from build123d import *

# Parameters (mm, degrees)
SKETCH1_W          = 12
SKETCH1_H          = 2.5
CHAMFER1_SIZE      = 0.6
CUT_EXTRUDE2_DEPTH = 1.925


with BuildPart() as part:
    # Sketch1 → Revolve1 (revolve)
    with BuildSketch(Plane(origin=(0, 0, 0), x_dir=(0, 0, -1), z_dir=(1, 0, 0))):
        with Locations((8.75, 1.25)):
            Rectangle(SKETCH1_W, SKETCH1_H)
    revolve(axis=Axis((0, 0, -14.75), (0, 0, 1)))

    # Chamfer1
    chamfer1_edges = [part.edges().sort_by_distance(p)[0] for p in [
        (0, -2.5, -14.75),
    ]]
    chamfer(chamfer1_edges, length=CHAMFER1_SIZE)

    # Sketch7 → Revolve2 (revolve)
    with BuildSketch(Plane(origin=(0, 0, 0), x_dir=(0, 0, -1), z_dir=(1, 0, 0)), mode=Mode.PRIVATE) as revolve2_sk:
        with BuildLine():
            Line((2.3375, 4.75), (2.75, 4.75))
            Line((2.75, 4.75), (2.75, 0))
            Line((2.75, 0), (0, 0))
            Line((0, 0), (0, 2.5))
            ThreePointArc((0, 2.5), (0.991875183, 3.808753282), (2.3375, 4.75))
        make_face()
    revolve(revolve2_sk.sketch.rotate(Axis((0, 0, 0), (0, 0, -1)), 180), axis=Axis((0, 0, 0), (0, 0, -1)))

    # Sketch5 → Cut-Extrude2 (cut)
    with BuildSketch(Plane.XY):
        Polygon((1.5, -0.866025404), (1.5, 0.866025404), (0, 1.732050808), (-1.5, 0.866025404), (-1.5, -0.866025404), (0, -1.732050808), align=None)
    extrude(amount=-CUT_EXTRUDE2_DEPTH, mode=Mode.SUBTRACT)

    # Cut-Extrude3 cone 1 section (on through the dimple's axis) → Cut-Extrude3 (revolve, cut)
    with BuildSketch(Plane(origin=(0, 0, 0), x_dir=(0, -1, 0), z_dir=(1, 0, 0))):
        Polygon((0, 0), (1.732050808, 0), (0, 1.732050808), align=None)
    revolve(axis=Axis((0, 0, 0), (0, 0, -1)), mode=Mode.SUBTRACT)


solid = part.part
For this review, take the finished solid that the model builds, in its own axes (mm). A direction names the side the tool comes from. Round coordinates to 2 decimals unless told otherwise and drop trailing zeros. Write each loop counter-clockwise with the first axis right and the second up, starting at its lowest first coordinate (ties: lowest second). Pieces come first, ordered by that corner, then holes. Notation, with made-up numbers: (43, 44.25) -> (63, 44.25) arc R33 cw to (63, 75.25) -> close; hole circle Ø11 at (-36.5, 41). An arc over 180 degrees is marked (long way). Use CSV: the item, a comma, the result in double quotes.
(1) For faces 4 (the face through (4.637, 1.03, -2.547)), 5 (the face through (0.761, 1.293, -0.949)), 6 (the face through (2, -2, -2.75)), list the 3-axis set-ups (+Z, -Z, +X, -X, +Y, -Y) from which the entire face can be reached by the end or side of a thin tool; tool diameter is ignored.
Computed values:
face 4,"+Z, -Z"
face 5,"+Z"
face 6,"-Z"
(2) Draft analysis for pull direction Y (two halves, no side actions). For faces 1 (the face through (0.74, -1.305, -0.949)), 2 (the face through (0, 0, -14.75)), 3 (the face through (2.44, -0.54, -8.53)), state which applies: +Y half, -Y half, draft (parallel to the pull), parting line (faces both ways), or undercut.
Computed values:
face 1,"undercut"
face 2,"draft"
face 3,"parting line"
(3) Clearance check with flat-ended pins moving along their axes: P1, Ø5, axis at x = -2, z = -6.5, coming from the +Y side; P2, Ø0.5, axis at y = 0, z = -1, coming from the +X side; P3, Ø0.9, axis at y = -0.5, z = -0.5, coming from the -X side. State where each tip first meets the part, or that it passes through.
Computed values:
P1,"y = 2.5"
P2,"x = 4.04"
P3,"x = -3.74"
(4) Consider section D-D, the plane y = -3.5. Give the boundary of the cut face in (x, z), plus the area to 3 significant figures.
Computed values:
outline,"(-3.21, -2.75) -> (3.21, -2.75) -> (3.21, -2.34) arc R3.96 ccw to (-3.21, -2.34) -> close"
area,"10.0 mm²"
(5) To check wall thickness, follow L1, parallel to X at y = 0, z = -14; L2, parallel to Z at x = -1.75, y = -2.5; L3, parallel to X at y = 0.75, z = -12. State the ranges of each line that lie inside material, in increasing order. Write a range as [from, to].
Computed values:
L1,"[-2.5, 2.5]"
L2,"[-2.75, -0.34]"
L3,"[-2.38, 2.38]"
(6) Consider section C-C, the plane z = -13.25. Give the boundary of the cut face in (x, y).
Computed values:
outline,"circle Ø5 at (0, 0)"
(7) Consider section B-B, the plane z = -1.5. Give the boundary of the cut face in (x, y).
Computed values:
outline,"circle Ø8.48 at (0, 0); hole (-1.5, -0.87) -> (0, -1.73) -> (1.5, -0.87) -> (1.5, 0.87) -> (0, 1.73) -> (-1.5, 0.87) -> close"
